Work out the finished part from the listing and answer in its coordinate system (mm). Coordinates: 2 decimals unless noted, no trailing zeros. Write each loop counter-clockwise with the first axis right and the second up, starting at its lowest first coordinate (ties: lowest second). Pieces come first, ordered by that corner, then holes. Notation, with made-up numbers: (-39.75, 51.25) - (5.25, 51.25) arc R15 ccw to (5.25, 55.25) - close; hole circle Ø10 at (61, 6.5). An arc over 180 degrees is marked (long way). Use one line per item in the form item = value. Start each with the question number.
Item 1: Given pin 1 (6 mm diameter, centred on x = 32, z = 2.5, fed in from -Y); pin 2 (4 mm diameter, centred on y = 88.5, z = 7.5, fed in from +X); pin 3 (2 mm diameter, centred on y = -78, z = 6.5, fed in from -X); pin 4 (1 mm diameter, centred on x = 58.5, y = 84, fed in from -Z), each flat-ended and moving along its own axis, determine where each tip first touches the part or whether it passes through.
Item 2: Consider probe 1 along Y at (x, z) = (31, 4.25); probe 2 along Y at (x, z) = (-16.5, 9); probe 3 along X at (y, z) = (85, 9.75). Determine where each line is inside the solid, lowest interval first.
Item 3: A cutting plane is placed at B-B (z = 5). Write down the section's boundary in (x, y).
from build123d import *

# Parameters (mm, degrees)
F1_DEPTH = 14
F2_SIZE2 = 8.082894
F2_SIZE  = 13.99999


# Not quite as in the source:
# - a fillet or chamfer is up to 0.001 mm smaller than in the source, because OpenCascade refuses the exact size


with BuildPart() as f1:
    # F0 (on Top) → F1 (new body)
    with BuildSketch(Plane.XY):
        Polygon((123.8743728424, -90), (123.8743728424, 90), (-47.3158000907, 145.6230589875), (-153.1171455034, 0), (-47.3158000907, -145.6230589875), align=None)
    extrude(amount=F1_DEPTH)

    # F2 (size 14 and 8.0829037687 in the source; OpenCascade refuses exactly that, so slightly less here)
    f2_edges = [f1.edges().sort_by_distance(p)[0] for p in [
        (38.279286, -117.811529, 14),
        (123.874373, 0, 14),
        (38.279286, 117.811529, 14),
        (-100.216473, 72.811529, 14),
        (-100.216473, -72.811529, 14),
    ]]
    chamfer(f2_edges, length=F2_SIZE, length2=F2_SIZE2)


with BuildPart() as f3_1:
    # F3: copy of F1
    add(f1.part)


with BuildPart() as f5_1:
    # F5: copy of F1
    add(f1.part.moved(Location((14, 14, 14))))


solid = f1.part
Answer:
q1.pin_1 = -120.39
q1.pin_2 = 120.58
q1.pin_3 = -92.83
q1.pin_4 = 0
q2.probe_1 = -117.6 to 117.6
q2.probe_2 = -130.15 to 130.15
q2.probe_3 = -84.4 to 118.25
q3.outline = (-149.55, 0) - (-46.21, -142.23) - (120.99, -87.9) - (120.99, 87.9) - (-46.21, 142.23) - close
